For this review, take the finished solid that the model builds, in its own axes (mm). Face numbers are marked on the shaded views. A direction names the side the tool comes from. Give positions to 0.01 mm unless a question says otherwise; leave off trailing zeros. Order: outer loops, then holes, each group sorted by start corner. A loop starts at its lowest first (then second) coordinate and runs counter-clockwise, first axis right, second up. Notation, with made-up numbers: (20.5, -36.75) - (57.5, -36.75) arc R5 ccw to (57.5, -27.75) - close; hole circle Ø2 at (79, 61.5). An arc over 180 degrees is marked (long way). Use a Markdown table: item, result. Add a question column.
1) We need section A-A on x = 0. Write out the cut boundary in (y, z), then the cut area to 3 significant figures.
2) We need section B-B on y = 9.5. Write out the cut boundary in (x, z), then the cut area to 3 significant figures.
3) Wall thickness on L1, parallel to Y at x = -7.5, z = 5; L2, parallel to Y at x = 0, z = 13.25; L3, parallel to Z at x = 0, y = -4.65: over which ranges is each line inside the solid? List them lowest first.
4) We need section D-D on z = 5. Write out the cut boundary in (x, y).
5) Clearance check with flat-ended pins moving along their axes: P1, Ø10, axis at x = 8.5, y = -9, coming from the +Z side; P2, Ø8, axis at y = 10, z = 3, coming from the -X side; P3, Ø1.9, axis at x = 6.72, y = 6.72, coming from the -Z side; P4, Ø2, axis at x = 3, z = 9.5, coming from the +Y side. State where each tip first meets the part, or that it passes through.
6) We need section C-C on z = 11. Write out the cut boundary in (x, y).
7) Mouldability with a two-part tool opening along Y and no side actions: class the marked faces 3, 4, 5 and 6 as released by +Y, released by -Y, zero draft, split by the parting line, or undercut.
8) Machinability: for the marked faces 1 and 2, which of the approach directions +Z, -Z, +X, -X, +Y, -Y give a long, thin tool a straight path to every point of the face, cutting with its end or side? Answer none if there is none.
```python
from build123d import *

# Parameters (mm, degrees)
SKETCH2_R               = 12.5
BOSS_EXTRUDE1_DEPTH     = 6
SKETCH3_R               = 6.5
SKETCH3_R_2             = 2.5
BOSS_EXTRUDE2_DEPTH     = 10
SKETCH4_R               = 1.2
CUT_EXTRUDE1_DEPTH      = 25
CUT_EXTRUDE1_DEPTH_BACK = 25
SKETCH5_R               = 1.2
CUT_EXTRUDE2_DEPTH      = 25
CIRPATTERN1_COUNT       = 2
CIRPATTERN1_ANGLE       = 45
SKETCH6_R               = 2.6
CUT_EXTRUDE3_DEPTH      = 50
CUT_EXTRUDE3_DEPTH_BACK = 20
CIRPATTERN2_COUNT       = 2
CIRPATTERN2_ANGLE       = 315
MIRROR1_COPY_1_SKETCH_R = 1.2
MIRROR1_COPY_1_DEPTH    = 25
MIRROR1_COPY_2_SKETCH_R = 1.2
MIRROR1_COPY_2_DEPTH    = 25


with BuildPart() as part:
    # Sketch2 → Boss-Extrude1 (new body)
    with BuildSketch(Plane.XY):
        Circle(SKETCH2_R)
    extrude(amount=BOSS_EXTRUDE1_DEPTH)

    # Sketch3 → Boss-Extrude2 (add)
    with BuildSketch(Plane.XY.offset(6)):
        Circle(SKETCH3_R)
        Circle(SKETCH3_R_2, mode=Mode.SUBTRACT)
    extrude(amount=BOSS_EXTRUDE2_DEPTH)

    # Sketch4 → Cut-Extrude1 (cut, two sides)
    with BuildSketch(Plane(origin=(0, 0, 0), x_dir=(1, 0, 0), z_dir=(0, 1, 0))) as cut_extrude1_sk:
        with Locations((0, -11)):
            Circle(SKETCH4_R)
    extrude(amount=CUT_EXTRUDE1_DEPTH, mode=Mode.SUBTRACT)
    extrude(cut_extrude1_sk.sketch, amount=-CUT_EXTRUDE1_DEPTH_BACK, mode=Mode.SUBTRACT)

    # Sketch5 → Cut-Extrude2 (cut, symmetric)
    with BuildSketch(Plane.XY.offset(6)):
        with Locations((0, 9.5)):
            Circle(SKETCH5_R)
    cut_extrude2 = extrude(amount=CUT_EXTRUDE2_DEPTH, both=True, mode=Mode.SUBTRACT)

    # CirPattern1: Cut-Extrude2 ×2 about axis
    cirpattern1_axis = Axis((0, 0, -0.6), (0, 0, 1))
    for i in range(1, CIRPATTERN1_COUNT):
        add(cut_extrude2.rotate(cirpattern1_axis, i * CIRPATTERN1_ANGLE / (CIRPATTERN1_COUNT - 1)), mode=Mode.SUBTRACT)

    # Sketch6 → Cut-Extrude3 (cut, two sides)
    with BuildSketch(Plane.XY.offset(6)) as cut_extrude3_sk:
        Circle(SKETCH6_R)
    extrude(amount=CUT_EXTRUDE3_DEPTH, mode=Mode.SUBTRACT)
    extrude(cut_extrude3_sk.sketch, amount=-CUT_EXTRUDE3_DEPTH_BACK, mode=Mode.SUBTRACT)

    # CirPattern2: Cut-Extrude2 ×2 about axis
    cirpattern2_axis = Axis((0, 0, 6), (0, 0, 1))
    for i in range(1, CIRPATTERN2_COUNT):
        add(cut_extrude2.rotate(cirpattern2_axis, i * CIRPATTERN2_ANGLE / (CIRPATTERN2_COUNT - 1)), mode=Mode.SUBTRACT)

    # Mirror1: Cut-Extrude2 across plane
    add(cut_extrude2.mirror(Plane.ZX), mode=Mode.SUBTRACT)

    # Mirror1 copy 1 sketch → Mirror1 copy 1 (cut, symmetric)
    with BuildSketch(Plane(origin=(0, 0, 6), x_dir=(0.707106781, 0.707106781, 0), z_dir=(0, 0, 1))):
        with Locations((0, -9.5)):
            Circle(MIRROR1_COPY_1_SKETCH_R)
    extrude(amount=MIRROR1_COPY_1_DEPTH, both=True, mode=Mode.SUBTRACT)

    # Mirror1 copy 2 sketch → Mirror1 copy 2 (cut, symmetric)
    with BuildSketch(Plane(origin=(0, 0, 6), x_dir=(0.707106781, -0.707106781, 0), z_dir=(0, 0, 1))):
        with Locations((0, -9.5)):
            Circle(MIRROR1_COPY_2_SKETCH_R)
    extrude(amount=MIRROR1_COPY_2_DEPTH, both=True, mode=Mode.SUBTRACT)


solid = part.part
```
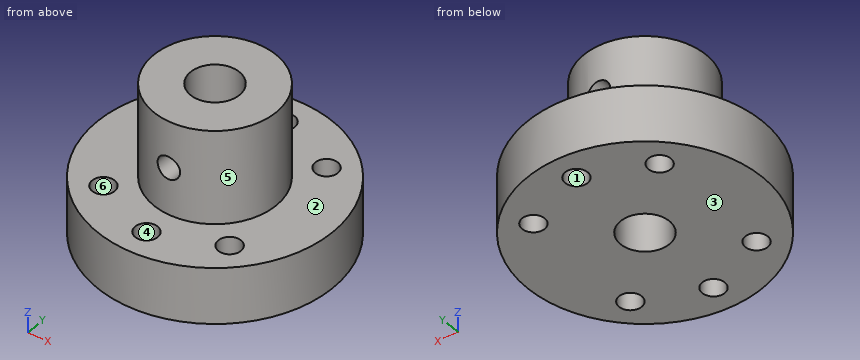
Checked values:
| question | item | result |
|---|---|---|
| 1 | outline | (-12.5, 0) - (-10.7, 0) - (-10.7, 6) - (-12.5, 6) - close; (-8.3, 0) - (-2.6, 0) - (-2.6, 9.8) - (-6.5, 9.8) - (-6.5, 6) - (-8.3, 6) - close; (-6.5, 12.2) - (-2.6, 12.2) - (-2.6, 16) - (-6.5, 16) - close; (2.6, 0) - (8.3, 0) - (8.3, 6) - (6.5, 6) - (6.5, 9.8) - (2.6, 9.8) - close; (2.6, 12.2) - (6.5, 12.2) - (6.5, 16) - (2.6, 16) - close; (10.7, 0) - (12.5, 0) - (12.5, 6) - (10.7, 6) - close |
| 1 | area | 149 mm² |
| 2 | outline | (-8.12, 0) - (-1.2, 0) - (-1.2, 6) - (-8.12, 6) - close; (1.2, 0) - (8.12, 0) - (8.12, 6) - (1.2, 6) - close |
| 2 | area | 83.1 mm² |
| 3 | L1 | -10 to -7.63, -5.81 to 5.81, 7.63 to 10 |
| 3 | L2 | -6.5 to -2.6, 2.6 to 6.5 |
| 3 | L3 | 0 to 9.8, 12.2 to 16 |
| 4 | outline | circle Ø25 at (0, 0); hole circle Ø2.4 at (-6.72, -6.72); hole circle Ø2.4 at (-6.72, 6.72); hole circle Ø5.2 at (0, 0); hole circle Ø2.4 at (0, -9.5); hole circle Ø2.4 at (0, 9.5); hole circle Ø2.4 at (6.72, -6.72); hole circle Ø2.4 at (6.72, 6.72) |
| 5 | P1 | z = 6 |
| 5 | P2 | x = -10.97 |
| 5 | P3 | through |
| 5 | P4 | y = 6.18 |
| 6 | outline | (-1.2, -6.39) - (-1.2, -2.31) arc R2.6 cw to (-1.2, 2.31) - (-1.2, 6.39) arc R6.5 ccw to start; (1.2, -6.39) arc R6.5 ccw to (1.2, 6.39) - (1.2, 2.31) arc R2.6 cw to (1.2, -2.31) - close |
| 7 | face 3 | zero draft |
| 7 | face 4 | undercut |
| 7 | face 5 | split by the parting line |
| 7 | face 6 | undercut |
| 8 | face 1 | +Z, -Z |
| 8 | face 2 | +Z |
